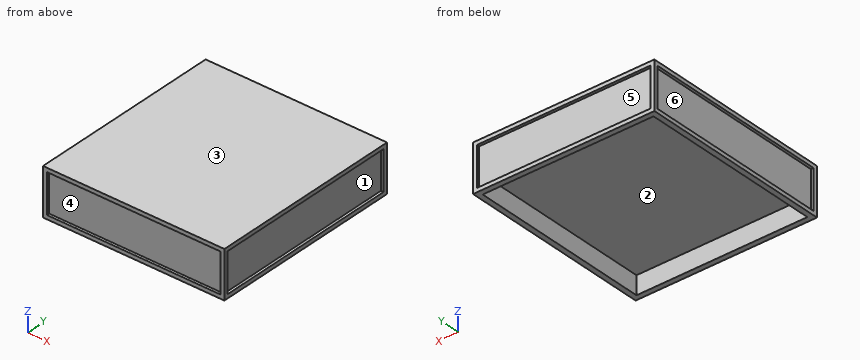
```python
from build123d import *

# Parameters (mm, degrees)
F0_W      = 690
F0_H      = 740
F1_DEPTH  = 180
F2_W      = 650
F2_H      = 700
F3_DEPTH  = 70
F5_W      = 710
F5_H      = 150
F8_DEPTH  = 10
F7_W      = 660
F7_H      = 150
F9_DEPTH  = 10
F6_W      = 710
F6_H      = 150
F10_DEPTH = 10
F4_W      = 660
F4_H      = 150
F11_DEPTH = 10


with BuildPart() as f1:
    # F0 (on Top) → F1 (new body)
    with BuildSketch(Plane.XY):
        Rectangle(F0_W, F0_H)
    extrude(amount=F1_DEPTH)

    # F2 (on face) → F3 (cut)
    with BuildSketch(Plane(origin=(0, 0, 0), x_dir=(1, 0, 0), z_dir=(0, 0, -1))):
        Rectangle(F2_W, F2_H)
    extrude(amount=-F3_DEPTH, mode=Mode.SUBTRACT)

    # F5 (on face) → F8 (cut)
    with BuildSketch(Plane.YZ.offset(345)):
        with Locations((0, 90)):
            Rectangle(F5_W, F5_H)
    extrude(amount=-F8_DEPTH, mode=Mode.SUBTRACT)

    # F7 (on face) → F9 (cut)
    with BuildSketch(Plane(origin=(0, 370, 0), x_dir=(-1, 0, 0), z_dir=(0, 1, 0))):
        with Locations((0, 90)):
            Rectangle(F7_W, F7_H)
    extrude(amount=-F9_DEPTH, mode=Mode.SUBTRACT)

    # F6 (on face) → F10 (cut)
    with BuildSketch(Plane(origin=(-345, 0, 0), x_dir=(0, -1, 0), z_dir=(-1, 0, 0))):
        with Locations((0, 90)):
            Rectangle(F6_W, F6_H)
    extrude(amount=-F10_DEPTH, mode=Mode.SUBTRACT)

    # F4 (on face) → F11 (cut)
    with BuildSketch(Plane.XZ.offset(370)):
        with Locations((0, 90)):
            Rectangle(F4_W, F4_H)
    extrude(amount=-F11_DEPTH, mode=Mode.SUBTRACT)


solid = f1.part
```
Check sheet for the modelled part. Datum: model origin and axes. Units: mm. Face numbers are marked on the shaded views. A direction names the side the tool comes from. Give positions to 0.01 mm unless a question says otherwise; leave off trailing zeros. Write each loop counter-clockwise with the first axis right and the second up, starting at its lowest first coordinate (ties: lowest second). Pieces come first, ordered by that corner, then holes. Notation, with made-up numbers: (35, -19) -> (58, -19) arc R28 ccw to (58, 3) -> close; hole circle Ø1 at (49, 88.25). An arc over 180 degrees is marked (long way). Use CSV: the item, a comma, the result in double quotes. Start each with the question number.
Q1. Depth check by flat-ended pin: P1, Ø1.5, axis at y = -207.5, z = 59.5, coming from the -X side; P2, Ø8, axis at x = 123, z = 123, coming from the -Y side; P3, Ø6, axis at y = -216, z = 131.5, coming from the +X side. Enter the tip coordinate at first touch or a pass-through.
Q2. Tool access check on the marked faces 1 and 2. Record the directions out of +Z, -Z, +X, -X, +Y, -Y that give a thin tool (end or side, any length) a straight path to the whole face; none if there is none.
Q3. Release check for a two-part mould opening along Y. For the marked faces 3, 4, 5 and 6 record: +Y half, -Y half, draft (parallel to the pull), parting line (faces both ways), or undercut.
Q4. Cross-section at A-A on z = 24. Enter the section's corners in (x, y), and give its area (3 significant figures).
Q5. Cross-section at B-B on x = -79.5. Enter the section's corners in (y, z), and give its area (3 significant figures).
Q6. Cross-section at C-C on y = 300. Enter the section's corners in (x, z).
Q7. Scan lines: line 1 along Y through (x, z) = (251, 14); line 2 along Y through (x, z) = (-126.5, 49); line 3 along X through (y, z) = (51, 60.5). Record each from-to range of solid material in increasing order.
Q8. Cross-section at D-D on z = 145. Enter the section's corners in (x, y).
Working result:
1,P1,"stops at x = -335"
1,P2,"stops at y = -360"
1,P3,"stops at x = 335"
2,face 1,"+X"
2,face 2,"-Z"
3,face 3,"draft"
3,face 4,"-Y half"
3,face 5,"+Y half"
3,face 6,"undercut"
4,outline,"(-345, -370) -> (-330, -370) -> (-330, -360) -> (330, -360) -> (330, -370) -> (345, -370) -> (345, -355) -> (335, -355) -> (335, 355) -> (345, 355) -> (345, 370) -> (330, 370) -> (330, 360) -> (-330, 360) -> (-330, 370) -> (-345, 370) -> (-345, 355) -> (-335, 355) -> (-335, -355) -> (-345, -355) -> close; hole (-325, -350) -> (325, -350) -> (325, 350) -> (-325, 350) -> close"
4,area,"28,200 mm^2"
5,outline,"(-370, 0) -> (-350, 0) -> (-350, 70) -> (350, 70) -> (350, 0) -> (370, 0) -> (370, 15) -> (360, 15) -> (360, 165) -> (370, 165) -> (370, 180) -> (-370, 180) -> (-370, 165) -> (-360, 165) -> (-360, 15) -> (-370, 15) -> close"
5,area,"81,200 mm^2"
6,outline,"(-345, 0) -> (-325, 0) -> (-325, 70) -> (325, 70) -> (325, 0) -> (345, 0) -> (345, 15) -> (335, 15) -> (335, 165) -> (345, 165) -> (345, 180) -> (-345, 180) -> (-345, 165) -> (-335, 165) -> (-335, 15) -> (-345, 15) -> close"
7,line 1,"y = -370 to -350, 350 to 370"
7,line 2,"y = -360 to -350, 350 to 360"
7,line 3,"x = -335 to -325, 325 to 335"
8,outline,"(-345, -370) -> (-330, -370) -> (-330, -360) -> (330, -360) -> (330, -370) -> (345, -370) -> (345, -355) -> (335, -355) -> (335, 355) -> (345, 355) -> (345, 370) -> (330, 370) -> (330, 360) -> (-330, 360) -> (-330, 370) -> (-345, 370) -> (-345, 355) -> (-335, 355) -> (-335, -355) -> (-345, -355) -> close"
